Geometry check sheet. Reference: the model listing, model coordinates, mm. A direction names the side the tool comes from. Round coordinates to 2 decimals unless told otherwise and drop trailing zeros. Write each loop counter-clockwise with the first axis right and the second up, starting at its lowest first coordinate (ties: lowest second). Pieces come first, ordered by that corner, then holes. Notation, with made-up numbers: (5, 52) -> (47, 52) arc R12 ccw to (47, 65) -> close; hole circle Ø3 at (56.5, 1). An arc over 180 degrees is marked (long way). Use a Markdown table: item, result.
Autodesk Inventor part; units mm, degrees
ref_plane "Work Plane1" through (0, 0, 1) normal (0, 0, 1) x (1, 0, 0)
ref_plane "Work Plane3" through (0, 0, 1) normal (0, 0, 1) x (1, 0, 0)
ref_plane "Work Plane2" through (0, 0, 1) normal (0, 0, 1) x (1, 0, 0)
sketch "Sketch1" plane through (0, 0, 0) normal (0, 0, 1) x (1, 0, 0)
  circle A0 centre (0, 0) radius 11.4
  dimension "d0" = 22.8
extrude "Extrusion1" add sketch "Sketch1" along normal blind 1
ref_plane "Work Plane1" through (0, 0, 1) normal (0, 0, 1) x (1, 0, 0)
sketch "Sketch3" plane through (0, 0, 1) normal (0, 0, 1) x (1, 0, 0)
  circle A0 centre (0, 0) radius 6.375
  circle A1 centre (0, 0) radius 5.375
  dimension "d6" = 12.75
  dimension "d7" = 10.75
extrude "Extrusion3" add sketch "Sketch3" along normal blind 2
ref_plane "Work Plane3" through (0, 0, 1) normal (0, 0, 1) x (1, 0, 0)
sketch "Sketch4" plane through (0, 0, 1) normal (0, 0, 1) x (1, 0, 0)
  circle A0 centre (0, 0) radius 1.425
  dimension "d10" = 2.85
extrude "Extrusion4" add sketch "Sketch4" along normal blind 24.1
ref_plane "Work Plane2" through (0, 0, 1) normal (0, 0, 1) x (1, 0, 0)
sketch "Sketch5" plane through (0, 0, 1) normal (0, 0, 1) x (1, 0, 0)
  circle A0 centre (0, 0) radius 4.125
  dimension "d14" = 8.25
extrude "Extrusion5" add sketch "Sketch5" along normal blind 0.4
sketch "Sketch7" plane through (0, 0, 1) normal (0, 0, 1) x (1, 0, 0)
  circle A0 centre (0, 0) radius 11.4
  line L0 (-1.1, 11.3468) -> (1.1, 11.3468) construction
  line L1 (0, 11.3468) -> (0, 10.5468) construction
  arc A1 (-1.1, 11.3468) -> (1.1, 11.3468) centre (0, 11.7031) ccw
  dimension "d17" = 2.2
  dimension "d18" = 0.8
extrude "Extrusion6" cut sketch "Sketch7" against normal up to surface (1 mm away) contours A1 A0 picked at (-0.044, 11.1142)
sketch "Sketch8" plane through (0, 0, 1) normal (0, 0, 1) x (1, 0, 0)
  arc A0 (-1.1, 11.3468) -> (1.1, 11.3468) centre (0, 11.7031) ccw
  arc A1 (-1.1, 11.3468) -> (1.1, 11.3468) centre (0, 0) ccw
  circle A2 centre (0, 0) radius 6.375
  arc A3 (-1.6146, 10.2739) -> (1.6146, 10.2739) centre (0, 11.7031) ccw
  arc A4 (-1.6146, 10.2739) -> (1.6146, 10.2739) centre (0, 0) ccw
  dimension "d21" = 1
extrude "Extrusion7" add sketch "Sketch8" along normal blind 0.57 contours A0 A1
properties part number "PMSeal"
(1) Section check D-D on z = 22. Record the cut outline in (x, y) (3 decimals).
A:
| item | result |
|---|---|
| outline | circle Ø2.85 at (0, 0) |
(2) Thickness scan on line 1 (Y direction, x = 0, z = 2.2) (3 decimals); line 2 (Z direction, x = 4.5, y = 1.5); line 3 (Y direction, x = -5.75, z = 1.5). Record the ranges inside material, lowest first.
A:
| item | result |
|---|---|
| line 1 | y = -6.375 to -5.375, -1.425 to 1.425, 5.375 to 6.375 |
| line 2 | z = 0 to 1 |
| line 3 | y = -9.84 to -8.67, -2.75 to 2.75, 8.67 to 9.84 |
(3) Section check C-C on z = 2. Record the cut outline in (x, y) (3 decimals), plus the area to 3 significant figures.
A:
| item | result |
|---|---|
| outline | circle Ø12.75 at (0, 0); circle Ø2.85 at (0, 0); hole circle Ø10.75 at (0, 0) |
| area | 43.3 mm2 |
(4) Section check B-B on x = 0. Record the cut outline in (y, z) (3 decimals).
A:
| item | result |
|---|---|
| outline | (-11.4, 0) -> (10.547, 0) -> (10.547, 1.57) -> (9.547, 1.57) -> (9.547, 1) -> (6.375, 1) -> (6.375, 3) -> (5.375, 3) -> (5.375, 1) -> (4.125, 1) -> (4.125, 1.4) -> (1.425, 1.4) -> (1.425, 25.1) -> (-1.425, 25.1) -> (-1.425, 1.4) -> (-4.125, 1.4) -> (-4.125, 1) -> (-5.375, 1) -> (-5.375, 3) -> (-6.375, 3) -> (-6.375, 1) -> (-10.4, 1) -> (-10.4, 1.57) -> (-11.4, 1.57) -> close |
(5) Section check A-A on y = 0. Record the cut outline in (x, z) (3 decimals), plus the area to 3 significant figures.
A:
| item | result |
|---|---|
| outline | (-11.4, 0) -> (11.4, 0) -> (11.4, 1.57) -> (10.4, 1.57) -> (10.4, 1) -> (6.375, 1) -> (6.375, 3) -> (5.375, 3) -> (5.375, 1) -> (4.125, 1) -> (4.125, 1.4) -> (1.425, 1.4) -> (1.425, 25.1) -> (-1.425, 25.1) -> (-1.425, 1.4) -> (-4.125, 1.4) -> (-4.125, 1) -> (-5.375, 1) -> (-5.375, 3) -> (-6.375, 3) -> (-6.375, 1) -> (-10.4, 1) -> (-10.4, 1.57) -> (-11.4, 1.57) -> close |
| area | 98.8 mm2 |
(6) Access from +Z, -Z, +X, -X, +Y, -Y to the whole of each face (thin tool, end or side, straight path). Record for faces 1 (the face through (0.02, 10.547, 0.774)), 2 (the face through (2, -4, 1)).
A:
| item | result |
|---|---|
| face 1 | +Z, -Z, +Y |
| face 2 | +Z |
(7) Release check for a two-part mould opening along X. For faces 3 (the face through (3.8, 1.6, 1.2)), 4 (the face through (0, 0, 25.1)) record: +X half, -X half, draft (parallel to the pull), parting line (faces both ways), or undercut.
A:
| item | result |
|---|---|
| face 3 | undercut |
| face 4 | draft |
(8) Gauge pin test, flat ends, axial feed: pin 1 Ø10 at (x, z) = (2, 17.5) entering from +Y (3 decimals); pin 2 Ø4 at (x, y) = (-4.5, -3.5) entering from +Z; pin 3 Ø10 at (y, z) = (3, 11) entering from +X (3 decimals). Record the tip position at first contact, or that the pin passes through.
A:
| item | result |
|---|---|
| pin 1 | stops at y = 1.425 |
| pin 2 | stops at z = 3 |
| pin 3 | stops at x = 1.425 |
